Part model, mm, in its own coordinate system. Face numbers are marked on the shaded views. Round coordinates to 2 decimals unless told otherwise and drop trailing zeros. Loops run counter-clockwise (first coordinate to the right, second up) from the corner with the lowest first, then second, coordinate; pieces in that order, holes last.
(1) Flat gauge pins, fed straight in: pin 1 (1 mm diameter, centred on x = 0, z = 1.5, fed in from +Y); pin 2 (2 mm diameter, centred on x = -23.5, z = 1.5, fed in from +Y) (3 decimals); pin 3 (2 mm diameter, centred on x = 22.5, z = 1, fed in from +Y). Where does each tip first touch, or does it go through?
(2) Cut at B-B on x = 0. List the corners of the cut face in (y, z).
(3) Cut at A-A on y = 0. List the corners of the cut face in (x, z), then the cut area to 3 significant figures.
(4) Mould opens along Y. For the marked faces 1, 2 and 3 say: +Y half, -Y half, draft (parallel to the pull), parting line (faces both ways), or undercut.
(5) Cut at C-C on z = 3.5. List the corners of the cut face in (x, y), then the cut area to 3 significant figures.
(6) Probe probe 1 along Y at (x, z) = (0, 0.95); probe 2 along X at (y, z) = (-8, 1.5); probe 3 along Z at (x, y) = (15.5, 10). List the from-to ranges inside material, lowest first.
from build123d import *

# Parameters (mm, degrees)
SKETCH_R        = 26.7
PAD_DEPTH       = 2
SKETCH001_W     = 5.2
SKETCH001_H     = 2.5
SKETCH001_W_2   = 2.5
SKETCH001_H_2   = 5.2
POCKET_DEPTH    = 2.001
SKETCH002_R     = 6
POCKET001_DEPTH = 2.001
SKETCH003_R     = 7.5
PAD001_DEPTH    = 4
SKETCH004_R     = 6
POCKET002_DEPTH = 1.001
SKETCH005_W     = 2
SKETCH005_H     = 2.479431
SKETCH005_H_2   = 2.486512
POCKET003_DEPTH = 1


with BuildPart() as part:
    # Sketch → Pad (new body)
    with BuildSketch(Plane.XY):
        Circle(SKETCH_R)
    extrude(amount=PAD_DEPTH)

    # Sketch001 → Pocket (cut, through all)
    with BuildSketch(Plane.XY.offset(2)):
        with Locations((-23.1, 0)):
            Rectangle(SKETCH001_W, SKETCH001_H)
        with Locations((23.1, 0)):
            Rectangle(SKETCH001_W, SKETCH001_H)
        with Locations((0, 23.1)):
            Rectangle(SKETCH001_W_2, SKETCH001_H_2)
        with Locations((0, -23.1)):
            Rectangle(SKETCH001_W_2, SKETCH001_H_2)
        Polygon((-19.029555, 17.261788), (-17.261788, 19.029555), (-13.584833, 15.3526), (-15.3526, 13.584833), align=None)
        Polygon((17.261788, 19.029555), (19.029555, 17.261788), (15.3526, 13.584833), (13.584833, 15.3526), align=None)
        Polygon((17.261788, -19.029555), (19.029555, -17.261788), (15.3526, -13.584833), (13.584833, -15.3526), align=None)
        Polygon((-17.261788, -19.029555), (-19.029555, -17.261788), (-15.3526, -13.584833), (-13.584833, -15.3526), align=None)
        Polygon((8.680115, 24.222058), (6.690161, 19.417885), (8.99986, 18.461176), (10.989814, 23.26535), align=None)
        Polygon((18.461176, 8.99986), (19.417885, 6.690161), (24.037282, 8.603578), (23.080574, 10.913277), align=None)
        Polygon((-23.26535, 10.989814), (-24.222058, 8.680115), (-19.417885, 6.690161), (-18.461176, 8.99986), align=None)
        Polygon((-24.222058, -8.680115), (-23.26535, -10.989814), (-18.461176, -8.99986), (-19.417885, -6.690161), align=None)
        Polygon((-10.989814, -23.26535), (-8.680115, -24.222058), (-6.690161, -19.417885), (-8.99986, -18.461176), align=None)
        Polygon((6.690161, -19.417885), (8.680115, -24.222058), (10.989814, -23.26535), (8.99986, -18.461176), align=None)
        Polygon((19.417885, -6.690161), (18.461176, -8.99986), (23.26535, -10.989814), (24.222058, -8.680115), align=None)
        Polygon((-10.989814, 23.26535), (-8.680115, 24.222058), (-6.690161, 19.417885), (-8.99986, 18.461176), align=None)
        Polygon((19.862235, 5.225333), (20.349961, 2.77337), (25.253888, 3.748822), (24.766162, 6.200785), align=None)
        Polygon((-25.253888, -3.748822), (-24.766162, -6.200785), (-19.862235, -5.225333), (-20.349961, -2.77337), align=None)
        Polygon((-24.962319, 6.239803), (-25.450045, 3.78784), (-20.349961, 2.77337), (-19.862235, 5.225333), align=None)
        Polygon((-20.764428, 15.182615), (-21.97311, 13.373695), (-17.649468, 10.48473), (-16.440786, 12.29365), align=None)
        Polygon((-14.45738, 19.861687), (-12.767282, 21.551783), (-9.972119, 17.651556), (-11.987236, 16.091467), align=None)
        Polygon((-5.876879, 24.541956), (-3.081719, 25.126991), (-2.366674, 18.561611), (-5.096836, 18.171587), align=None)
        Polygon((3.873685, 24.60696), (2.70362, 19.666674), (4.523721, 19.146645), (6.148817, 23.891918), align=None)
        Polygon((12.714202, 21.031754), (9.659025, 16.416485), (11.609138, 15.311421), (14.339291, 19.406658), align=None)
        Polygon((16.350664, 12.428527), (17.73959, 10.349853), (22.063232, 13.238818), (20.674306, 15.317492), align=None)
        Polygon((20.349961, -2.77337), (19.862235, -5.225333), (24.962319, -6.239803), (25.450045, -3.78784), align=None)
        Polygon((17.649468, -10.48473), (16.440786, -12.29365), (20.764428, -15.182615), (21.97311, -13.373695), align=None)
        Polygon((11.154702, -18.639545), (12.909801, -17.534479), (14.534897, -20.524654), (12.779791, -22.019741), align=None)
        Polygon((2.379186, -20.914677), (5.239352, -20.264639), (6.344416, -24.554888), (3.679265, -25.334934), align=None)
        Polygon((-2.756109, -21.629719), (-3.536156, -25.26993), (-6.201311, -24.489885), (-5.291257, -20.849672), align=None)
        Polygon((-14.651802, -20.199635), (-13.026706, -21.369703), (-10.296549, -17.144459), (-12.246662, -16.234406), align=None)
        Polygon((-22.063232, -13.238818), (-20.674306, -15.317492), (-16.350664, -12.428527), (-17.73959, -10.349853), align=None)
    extrude(amount=-POCKET_DEPTH, mode=Mode.SUBTRACT)

    # Sketch002 → Pocket001 (cut, through all)
    with BuildSketch(Plane.XY.offset(2)):
        Circle(SKETCH002_R)
    extrude(amount=-POCKET001_DEPTH, mode=Mode.SUBTRACT)

    # Sketch003 → Pad001 (new body)
    with BuildSketch(Plane.XY.offset(2)):
        Circle(SKETCH003_R)
    extrude(amount=PAD001_DEPTH)

    # Sketch004 → Pocket002 (cut, through all)
    with BuildSketch(Plane.XZ.offset(-25.7)):
        Circle(SKETCH004_R)
    extrude(amount=-POCKET002_DEPTH, mode=Mode.SUBTRACT)

    # Sketch005 → Pocket003 (cut)
    with BuildSketch(Plane(origin=(0, 25.7, 0), x_dir=(-1, 0, 0), z_dir=(0, 1, 0))):
        with Locations((0, -6.731688)):
            Rectangle(SKETCH005_W, SKETCH005_H)
        with Locations((0, 6.735229)):
            Rectangle(SKETCH005_W, SKETCH005_H_2)
    extrude(amount=-POCKET003_DEPTH, mode=Mode.SUBTRACT)


solid = part.part
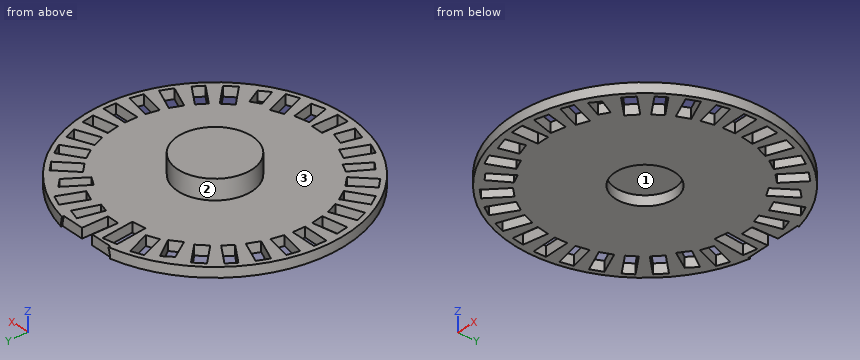
Final values:
1. pin 1: stops at y = 20.5
1. pin 2: stops at y = 14.375
1. pin 3: stops at y = 15.83
2. outline: (-26.7, 0) - (-25.7, 0) - (-25.7, 2) - (-26.7, 2) - close; (-20.5, 0) - (-6, 0) - (-6, 2) - (6, 2) - (6, 0) - (20.5, 0) - (20.5, 2) - (7.5, 2) - (7.5, 6) - (-7.5, 6) - (-7.5, 2) - (-20.5, 2) - close
3. outline: (-26.7, 0) - (-25.7, 0) - (-25.7, 2) - (-26.7, 2) - close; (-20.5, 0) - (-6, 0) - (-6, 2) - (6, 2) - (6, 0) - (20.5, 0) - (20.5, 2) - (7.5, 2) - (7.5, 6) - (-7.5, 6) - (-7.5, 2) - (-20.5, 2) - close; (25.7, 0) - (26.7, 0) - (26.7, 2) - (25.7, 2) - close
3. area: 122 mm2
4. face 1: undercut
4. face 2: parting line
4. face 3: draft
5. outline: circle Ø15 at (0, 0)
5. area: 177 mm2
6. probe 1: y = -26.7 to -25.7, -20.5 to -6, 6 to 20.5
6. probe 2: x = -25.47 to -22.58, -18.88 to 18.88, 22.58 to 25.47
6. probe 3: z = 0 to 2
